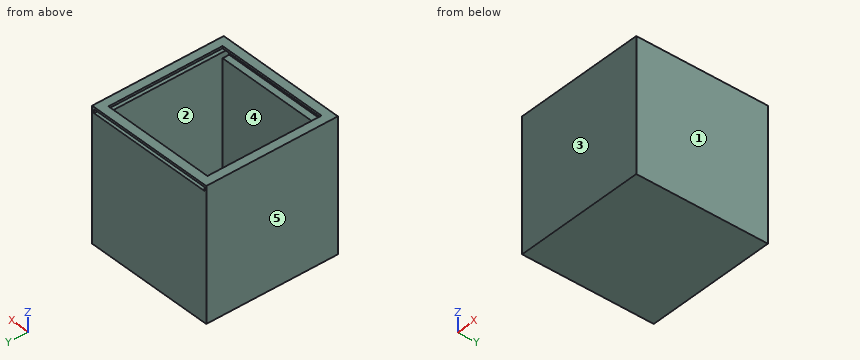
```python
from build123d import *

# Parameters (mm, degrees)
F0_W     = 76.2
F0_H     = 76.2
F1_DEPTH = 76.2
F2_T     = -5.08
F3_W     = 73.6691647935
F3_H     = 2.159
F4_DEPTH = 74.93
F5_W     = 66.04
F5_H     = 5.4402127862
F6_DEPTH = 3.81
F7_W     = 3.81
F7_H     = 2.159
F7_W_2   = 3.8191647935
F8_DEPTH = 1.905


with BuildPart() as f1:
    # F0 (on Top) → F1 (new body)
    with BuildSketch(Plane.XY):
        Rectangle(F0_W, F0_H)
    extrude(amount=F1_DEPTH)

    # F2
    f2_openings = [f1.faces().sort_by_distance(p)[0] for p in [
        (0, 0, 76.2),
    ]]
    offset(amount=F2_T, openings=f2_openings)

    # F3 (on face) → F4 (cut)
    with BuildSketch(Plane(origin=(0, 38.1, 0), x_dir=(-1, 0, 0), z_dir=(0, 1, 0))):
        with Locations((0.0045823967, 73.8505)):
            Rectangle(F3_W, F3_H)
    extrude(amount=-F4_DEPTH, mode=Mode.SUBTRACT)

    # F5 (on face) → F6 (cut)
    with BuildSketch(Plane(origin=(0, -33.02, 0), x_dir=(-1, 0, 0), z_dir=(0, 1, 0))):
        with Locations((0, 72.1777938306)):
            Rectangle(F5_W, F5_H)
    extrude(amount=-F6_DEPTH, mode=Mode.SUBTRACT)

    # F7 (on face) → F8 (join)
    with BuildSketch(Plane(origin=(0, -36.83, 0), x_dir=(-1, 0, 0), z_dir=(0, 1, 0))):
        with Locations((-34.925, 73.8505)):
            Rectangle(F7_W, F7_H)
        with Locations((34.9295823967, 73.8505)):
            Rectangle(F7_W_2, F7_H)
    extrude(amount=F8_DEPTH)


solid = f1.part
```
Can you work these out from the model? Positions are in its coordinate system, mm. Face numbers are marked on the shaded views. A direction names the side the tool comes from. Round coordinates to 2 decimals unless told otherwise and drop trailing zeros. Loops run counter-clockwise (first coordinate to the right, second up) from the corner with the lowest first, then second, coordinate; pieces in that order, holes last. Notation, with made-up numbers: M 30,11.25 L 58,11.25 A30 cw 58,43.25 Z; hole C -36.75,1.25 d8. An arc over 180 degrees is marked long. Write item = value, one per line. Start each with the question number.
(1) Suppose I cut it at B-B on z = 33. Write out the boundary of the cut face in (x, y), plus the area to 3 significant figures.
(2) Suppose I cut it at A-A on x = 24. Write out the boundary of the cut face in (y, z).
(3) Which directions (+Z, -Z, +X, -X, +Y, -Y) give clear straight access to the entire face, cutting with the end or side of a thin tool? Please do the marked faces 4 and 5.
(4) I'm going to push flat-ended pins straight in: P1, Ø8, axis at x = -16, y = -26.5, coming from the +Z side; P2, Ø1.1, axis at x = 35.5, z = 74, coming from the +Y side (3 decimals). Where does each tip first touch, or does it pass through?
(5) If we mould it in two halves opening along Y, with no side actions, what happens to the marked faces 1, 2 and 3? For each: released by +Y, released by -Y, zero draft, split by the parting line, or undercut.
(6) Suppose I cut it at C-C on y = 2. Write out the boundary of the cut face in (x, z), plus the area to 3 significant figures.
(7) I need wall thicknesses on line 1 along X through (y, z) = (24.5, 48); line 2 along Z through (x, y) = (-27.5, -30). Which ranges of each line are inside material? Lowest first, please.
Answer block:
q1.outline = M -38.1,-38.1 L 38.1,-38.1 L 38.1,38.1 L -38.1,38.1 Z; hole M -33.02,-33.02 L 33.02,-33.02 L 33.02,33.02 L -33.02,33.02 Z
q1.area = 1,450 mm²
q2.outline = M -38.1,0 L 38.1,0 L 38.1,72.77 L 33.02,72.77 L 33.02,5.08 L -33.02,5.08 L -33.02,69.46 L -36.83,69.46 L -36.83,74.93 L -33.02,74.93 L -33.02,76.2 L -38.1,76.2 Z; M 33.02,74.93 L 38.1,74.93 L 38.1,76.2 L 33.02,76.2 Z
q3.face_4 = +Z
q3.face_5 = +Z, -Z, -X, +Y, -Y
q4.P1 = 5.08
q4.P2 = -34.925
q5.face_1 = zero draft
q5.face_2 = undercut
q5.face_3 = released by -Y
q6.outline = M -38.1,0 L 38.1,0 L 38.1,76.2 L 33.02,76.2 L 33.02,74.93 L 36.83,74.93 L 36.83,72.77 L 33.02,72.77 L 33.02,5.08 L -33.02,5.08 L -33.02,72.77 L -36.84,72.77 L -36.84,74.93 L -33.02,74.93 L -33.02,76.2 L -38.1,76.2 Z
q6.area = 1,090 mm²
q7.line_1 = -38.1 to -33.02, 33.02 to 38.1
q7.line_2 = 0 to 5.08
